from build123d import *

# Parameters (mm, degrees)
SKETCH1_R           = 6.35
BOSS_EXTRUDE1_DEPTH = 50.8
BOSS_EXTRUDE2_START = -3.175
SKETCH2_R           = 63.5
SKETCH2_R_2         = 60.325
BOSS_EXTRUDE2_DEPTH = 3.175
SKETCH6_R           = 63.5
SKETCH6_R_2         = 60.325
BOSS_EXTRUDE3_DEPTH = 3.175
SKETCH1_3_R         = 6.35
CUT_EXTRUDE1_DEPTH  = 50.8


with BuildPart() as part:
    # Sketch1 → Boss-Extrude1 (new body)
    with BuildSketch(Plane.XY):
        Circle(SKETCH1_R)
        with BuildLine():
            Line((59.700240967, -21.63634046), (25.336398074, -1.796366515))
            ThreePointArc((25.336398074, -1.796366515), (-25.399970938, -0.03842333), (25.330847289, 1.873012441))
            Line((25.330847289, 1.873012441), (60.726284541, -18.562552784))
            ThreePointArc((60.726284541, -18.562552784), (60.232873534, -20.105992785), (59.700240967, -21.63634046))
        make_face()
        with BuildLine():
            Line((26.915242167, -57.513648286), (16.645315944, -19.185761833))
            ThreePointArc((16.645315944, -19.185761833), (-17.987661089, 17.933322295), (19.23603369, -16.587194093))
            Line((19.23603369, -16.587194093), (29.814260645, -56.065674545))
            ThreePointArc((29.814260645, -56.065674545), (28.373989485, -56.808157167), (26.915242167, -57.513648286))
        make_face()
        with BuildLine():
            Line((-21.63634046, -59.700240967), (-1.796366515, -25.336398074))
            ThreePointArc((-1.796366515, -25.336398074), (-0.03842333, 25.399970938), (1.873012441, -25.330847289))
            Line((1.873012441, -25.330847289), (-18.562552784, -60.726284541))
            ThreePointArc((-18.562552784, -60.726284541), (-20.105992785, -60.232873534), (-21.63634046, -59.700240967))
        make_face()
        with BuildLine():
            Line((-57.513648286, -26.915242167), (-19.185761833, -16.645315944))
            ThreePointArc((-19.185761833, -16.645315944), (17.933322295, 17.987661089), (-16.587194093, -19.23603369))
            Line((-16.587194093, -19.23603369), (-56.065674545, -29.814260645))
            ThreePointArc((-56.065674545, -29.814260645), (-56.808157167, -28.373989485), (-57.513648286, -26.915242167))
        make_face()
        with BuildLine():
            Line((-59.700240967, 21.63634046), (-25.336398074, 1.796366515))
            ThreePointArc((-25.336398074, 1.796366515), (25.399970938, 0.03842333), (-25.330847289, -1.873012441))
            Line((-25.330847289, -1.873012441), (-60.726284541, 18.562552784))
            ThreePointArc((-60.726284541, 18.562552784), (-60.232873534, 20.105992785), (-59.700240967, 21.63634046))
        make_face()
        with BuildLine():
            Line((-26.915242167, 57.513648286), (-16.645315944, 19.185761833))
            ThreePointArc((-16.645315944, 19.185761833), (17.987661089, -17.933322295), (-19.23603369, 16.587194093))
            Line((-19.23603369, 16.587194093), (-29.814260645, 56.065674545))
            ThreePointArc((-29.814260645, 56.065674545), (-28.373989485, 56.808157167), (-26.915242167, 57.513648286))
        make_face()
        with BuildLine():
            Line((21.63634046, 59.700240967), (1.796366515, 25.336398074))
            ThreePointArc((1.796366515, 25.336398074), (0.03842333, -25.399970938), (-1.873012441, 25.330847289))
            Line((-1.873012441, 25.330847289), (18.562552784, 60.726284541))
            ThreePointArc((18.562552784, 60.726284541), (20.105992785, 60.232873534), (21.63634046, 59.700240967))
        make_face()
        with BuildLine():
            Line((57.513648286, 26.915242167), (19.185761833, 16.645315944))
            ThreePointArc((19.185761833, 16.645315944), (-17.933322295, -17.987661089), (16.587194093, 19.23603369))
            Line((16.587194093, 19.23603369), (56.065674545, 29.814260645))
            ThreePointArc((56.065674545, 29.814260645), (56.808157167, 28.373989485), (57.513648286, 26.915242167))
        make_face()
    extrude(amount=BOSS_EXTRUDE1_DEPTH)

    # Sketch2 → Boss-Extrude2 (add)
    with BuildSketch(Plane.XY.offset(50.8).offset(BOSS_EXTRUDE2_START)):
        with Locations(Location((0, 0, 0), (0, 0, 163.002878163))):
            Circle(SKETCH2_R)
        Circle(SKETCH2_R_2, mode=Mode.SUBTRACT)
    extrude(amount=BOSS_EXTRUDE2_DEPTH)

    # Sketch6 → Boss-Extrude3 (add)
    with BuildSketch(Plane(origin=(0, 0, 0), x_dir=(-1, 0, 0), z_dir=(0, 0, -1))):
        with Locations(Location((0, 0, 0), (0, 0, 180))):
            Circle(SKETCH6_R)
        Circle(SKETCH6_R_2, mode=Mode.SUBTRACT)
    extrude(amount=-BOSS_EXTRUDE3_DEPTH)

    # Sketch1<3> → Cut-Extrude1 (cut)
    with BuildSketch(Plane.XY):
        Circle(SKETCH1_3_R)
    extrude(amount=CUT_EXTRUDE1_DEPTH, mode=Mode.SUBTRACT)


solid = part.part
Work out the finished part from the listing and answer in its coordinate system (mm). Give positions to 0.01 mm unless a question says otherwise; leave off trailing zeros. Write each loop counter-clockwise with the first axis right and the second up, starting at its lowest first coordinate (ties: lowest second). Pieces come first, ordered by that corner, then holes. Notation, with made-up numbers: (-31, -15.75) - (-4, -15.75) arc R22 ccw to (-4, 4.25) - close; hole circle Ø5 at (73.25, 22). An arc over 180 degrees is marked (long way). One line per item, written item: value. Start each with the question number.
1. Consider probe 1 along Z at (x, y) = (-35.5, -51.5) (3 decimals); probe 2 along Y at (x, z) = (3, 29.5); probe 3 along Y at (x, z) = (0, 16) (3 decimals). Determine where each line is inside the solid, lowest interval first.
2. Given pin 1 (1.5 mm diameter, centred on y = 27.5, z = 12, fed in from +X); pin 2 (24.5 mm diameter, centred on x = -33.5, y = -45.5, fed in from -Z); pin 3 (6 mm diameter, centred on y = -10.5, z = 14.5, fed in from +X); pin 4 (10 mm diameter, centred on y = -29.5, z = 35.5, fed in from +X), each flat-ended and moving along its own axis, determine where each tip first touches the part or whether it passes through.
3. For a pull along Z with two mould halves and no side action, classify faces 1 (the flat face through (-4, 61, 3.175)), 2 (the cylindrical face through (-1.38, -6.2, 25.04)) as +Z half, -Z half, draft (parallel to the pull), parting line (faces both ways), or undercut.
4. Find section C-C (y = 35). Write down the section's boundary in (x, z) (3 decimals).
5. Find section B-B (x = -11.5). Write down the section's boundary in (y, z) (3 decimals).
Geometry results:
1. probe 1: 0 to 3.175, 47.625 to 50.8
1. probe 2: -25.22 to -5.6, 5.6 to 25.22, 27.42 to 33.77
1. probe 3: -28.575 to -6.35, 6.35 to 28.575
2. pin 1: x = 57.51
2. pin 2: z = 0
2. pin 3: x = 51.96
2. pin 4: x = 24.04
3. face 1: undercut
3. face 2: draft
4. outline: (-52.983, 0) - (-49.134, 0) - (-49.134, 3.175) - (-52.983, 3.175) - close; (-52.983, 47.625) - (-49.134, 47.625) - (-49.134, 50.8) - (-52.983, 50.8) - close; (-24.17, 0) - (-20.883, 0) - (-20.883, 50.8) - (-24.17, 50.8) - close; (3.709, 0) - (7.376, 0) - (7.376, 50.8) - (3.709, 50.8) - close; (49.134, 0) - (52.983, 0) - (52.983, 3.175) - (49.134, 3.175) - close; (49.134, 47.625) - (52.983, 47.625) - (52.983, 50.8) - (49.134, 50.8) - close
5. outline: (-62.45, 0) - (-59.219, 0) - (-59.219, 3.175) - (-62.45, 3.175) - close; (-62.45, 47.625) - (-59.219, 47.625) - (-59.219, 50.8) - (-62.45, 50.8) - close; (-48.494, 0) - (-42.144, 0) - (-42.144, 50.8) - (-48.494, 50.8) - close; (-22.648, 0) - (22.648, 0) - (22.648, 50.8) - (-22.648, 50.8) - close; (59.219, 0) - (62.45, 0) - (62.45, 3.175) - (59.219, 3.175) - close; (59.219, 47.625) - (62.45, 47.625) - (62.45, 50.8) - (59.219, 50.8) - close
